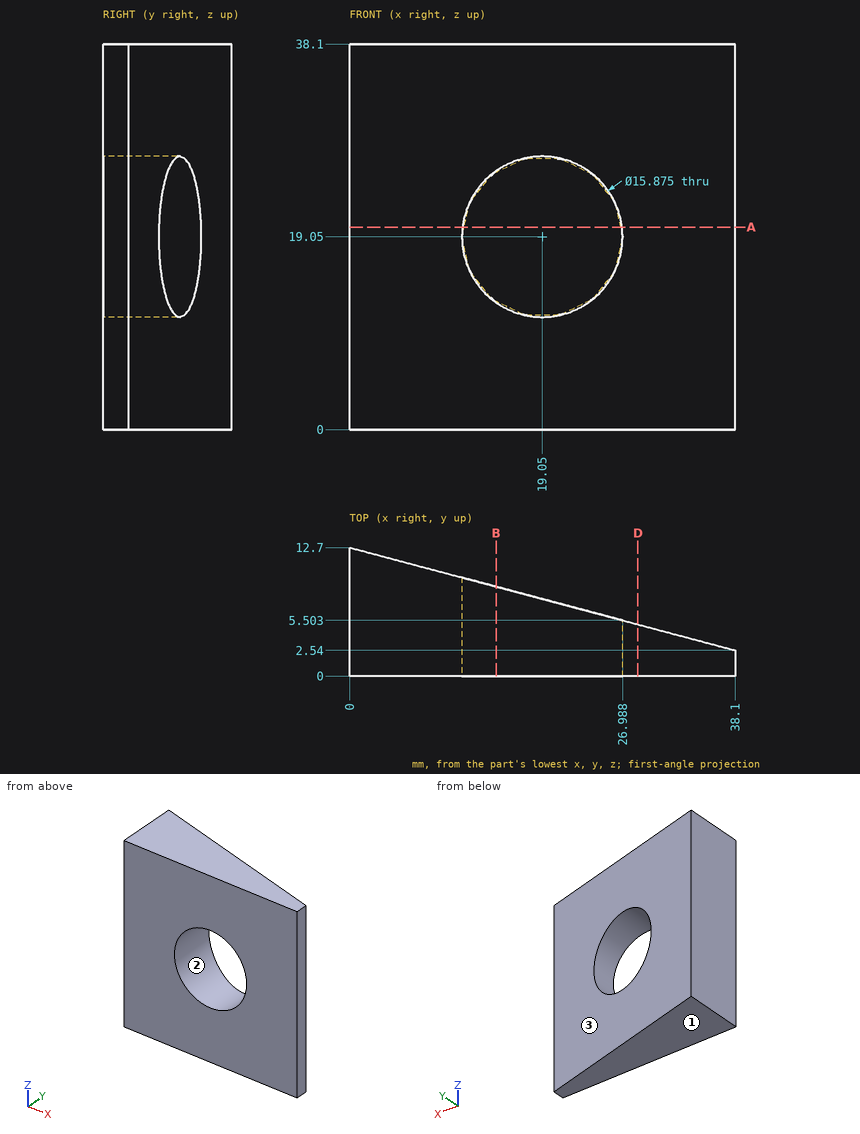
Print and shaded views of the part. All mm, measured from the part's lowest x, y and z. Round coordinates to 2 decimals unless told otherwise and drop trailing zeros. Write each loop counter-clockwise with the first axis right and the second up, starting at its lowest first coordinate (ties: lowest second). Pieces come first, ordered by that corner, then holes.
(1) Drop flat-ended pins along their axis: P1, Ø1.5, axis at x = 28.5, z = 11, coming from the +Y side; P2, Ø4, axis at x = 12.5, z = 5.5, coming from the +Y side. Give the stop position or say it passes through.
(2) Slice it at A-A, the plane z = 20. Write the cut outline in (x, y), and give its area (3 significant figures).
(3) Probe line 1 along Z through (x, y) = (19.05, 7); line 2 along Z through (x, y) = (20.5, 3.25) (1 decimal); line 3 along X through (y, z) = (6, 19.05). List the from-to ranges inside material, lowest first.
(4) Slice it at D-D, the plane x = 28.5. Write the cut outline in (y, z).
(5) Mould opens along Z. For the marked faces 1, 2 and 3 say: pulls with the +Z half, pulls with the -Z half, needs draft (parallel to the pull), parting line crosses it, or undercut.
(6) Slice it at B-B, the plane x = 14.5. Write the cut outline in (y, z), and give its area (3 significant figures).
From the geometry:
1. P1: stops at y = 5.3
1. P2: stops at y = 9.9
2. outline: (0, 0) - (11.17, 0) - (11.17, 9.72) - (0, 12.7) - close; (26.93, 0) - (38.1, 0) - (38.1, 2.54) - (26.93, 5.52) - close
2. area: 170 mm2
3. line 1: z = 0 to 11.11, 26.99 to 38.1
3. line 2: z = 0 to 11.2, 26.9 to 38.1
3. line 3: x = 0 to 11.11
4. outline: (0, 0) - (5.1, 0) - (5.1, 38.1) - (0, 38.1) - close
5. face 1: pulls with the -Z half
5. face 2: undercut
5. face 3: needs draft
6. outline: (0, 0) - (8.83, 0) - (8.83, 12.55) - (0, 12.55) - close; (0, 25.55) - (8.83, 25.55) - (8.83, 38.1) - (0, 38.1) - close
6. area: 222 mm2
